```python
from build123d import *
from build123d.topology import SkipClean

# Parameters (mm, degrees)
BOSS_EXTRUDE1_DEPTH     = 1.5
SKETCH2_R               = 3.5
BOSS_EXTRUDE2_DEPTH     = 2.3
CUT_EXTRUDE1_DEPTH      = 17.539044712
CUT_EXTRUDE1_DEPTH_BACK = 17.539044712
SKETCH3_R               = 0.375
SKETCH3_R_2             = 1.25


with BuildPart() as part:
    # Sketch1 → Boss-Extrude1 (new body)
    with BuildSketch(Plane(origin=(0, 0, 0), x_dir=(1, 0, 0), z_dir=(0, 1, 0))):
        with BuildLine():
            Line((2.257072219, 2.675), (14.110649579, 2))
            ThreePointArc((14.110649579, 2), (16, 0), (14.110649579, -2))
            Line((14.110649579, -2), (2.257072219, -2.675))
            ThreePointArc((2.257072219, -2.675), (-3.5, 0), (2.257072219, 2.675))
        make_face()
    extrude(amount=BOSS_EXTRUDE1_DEPTH)

    # Sketch2 → Boss-Extrude2 (add)
    with SkipClean():  # the faces are left unmerged after this step: merging them gives an invalid solid
        with BuildSketch(Plane(origin=(0, 1.5, 0), x_dir=(1, 0, 0), z_dir=(0, 1, 0))):
            with Locations(Location((0, 0, 0), (0, 0, 49.843487791))):
                Circle(SKETCH2_R)
        extrude(amount=BOSS_EXTRUDE2_DEPTH)

    # Sketch3 → Cut-Extrude1 (cut, two sides: drawn at the far end of the back side and taken through both)
    with SkipClean():  # the faces are left unmerged after this step: merging them gives an invalid solid
        with BuildSketch(Plane(origin=(0, 1.5, 0), x_dir=(1, 0, 0), z_dir=(0, 1, 0)).offset(-CUT_EXTRUDE1_DEPTH_BACK)):
            with Locations(Location((4.5, 0, 0), (0, 0, 270))):
                Circle(SKETCH3_R)
            with Locations(Location((0, 0, 0), (0, 0, 270))):
                Circle(SKETCH3_R_2)
            with Locations(Location((6.5, 0, 0), (0, 0, 270))):
                Circle(SKETCH3_R)
            with Locations(Location((8.5, 0, 0), (0, 0, 270))):
                Circle(SKETCH3_R)
            with Locations(Location((10.5, 0, 0), (0, 0, 270))):
                Circle(SKETCH3_R)
            with Locations(Location((12.5, 0, 0), (0, 0, 270))):
                Circle(SKETCH3_R)
            with Locations(Location((14.5, 0, 0), (0, 0, 270))):
                Circle(SKETCH3_R)
        extrude(amount=CUT_EXTRUDE1_DEPTH + CUT_EXTRUDE1_DEPTH_BACK, mode=Mode.SUBTRACT)


solid = part.part
```
Input: part model. Units: mm. Frame: model coordinates. Give positions to 0.01 mm unless a question says otherwise; leave off trailing zeros. Order: outer loops, then holes, each group sorted by start corner. A loop starts at its lowest first (then second) coordinate and runs counter-clockwise, first axis right, second up. Notation, with made-up numbers: M 64,4.25 L 74,4.25 A32 cw 74,34.25 Z; hole C -16,72.5 d6. An arc over 180 degrees is marked long. One line per question, with ' | ' between items. Start each with the question number.
1. Pull-direction query (X, two-part tool) for faces 1 (the face through (-1.22, 1.87, -0.27)), 2 (the face through (9.2, 1.5, 0)), 3 (the face through (16, 1, 0)); classes: released by +X, released by -X, zero draft, split by the parting line, or undercut.
2. Section query A-A (x = 0). Return the cut outline in (y, z).
3. Material intervals for probe 1 along Z at (x, y) = (0, 1.7); probe 2 along Y at (x, z) = (3.25, 2.25); probe 3 along X at (y, z) = (0.7, 1), sorted ascending. Write a range as [from, to].
4. Section query B-B (y = 1.1). Return the cut outline in (x, z) (3 decimals).
5. Section query C-C (z = 0). Count the separate pieces of the cut face and the enclosed holes in it, and give its area (3 significant figures).
6. Section query D-D (y = 2.4). Return the cut outline in (x, z) (3 decimals), and give its area (3 significant figures).
7. First-contact query: pin 1 Ø2 at (x, z) = (0, 0) entering from -Y; pin 2 Ø2 at (x, y) = (-1.5, 2) entering from -Z; pin 3 Ø4 at (x, z) = (7, 2) entering from +Y. Flat tips, straight axial feed; report the tip coordinate or a pass-through.
Here are the results:
1) face 1: undercut | face 2: zero draft | face 3: released by +X
2) outline: M 0,-3.5 L 3.8,-3.5 L 3.8,-1.25 L 0,-1.25 Z; M 0,1.25 L 3.8,1.25 L 3.8,3.5 L 0,3.5 Z
3) probe 1: [-3.5, -1.25], [1.25, 3.5] | probe 2: [0, 1.5] | probe 3: [-3.35, -0.75], [0.75, 15.73]
4) outline: M 2.257,-2.675 L 14.111,-2 A2.003 ccw 14.111,2 L 2.257,2.675 A3.5 ccw long Z; hole C 0,0 d2.5; hole C 4.5,0 d0.75; hole C 6.5,0 d0.75; hole C 8.5,0 d0.75; hole C 10.5,0 d0.75; hole C 12.5,0 d0.75; hole C 14.5,0 d0.75
5) separate pieces: 8 | enclosed holes: 0 | area: 29.1 mm²
6) outline: C 0,0 d7; hole C 0,0 d2.5 | area: 33.6 mm²
7) pin 1: through | pin 2: z = -3.46 | pin 3: y = 1.5
